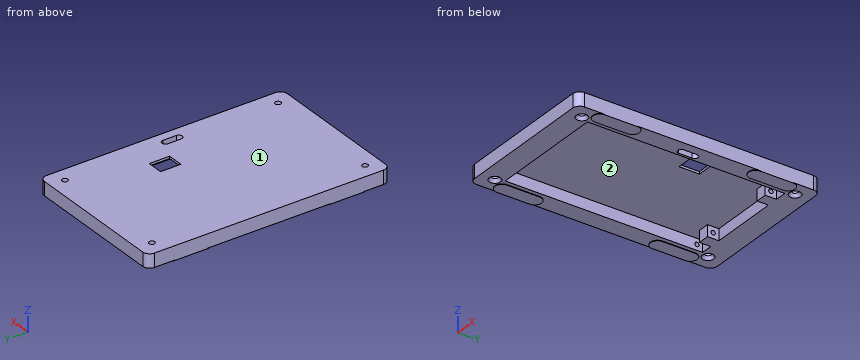
```python
from build123d import *

# Parameters (mm, degrees)
SKICA1_W                 = 67
SKICA1_H                 = 107
P_IDAT_VYSUNUT_M1_DEPTH  = 6
ZAOBLIT1_R               = 3
SKICA2_R                 = 1.25
ODEBRAT_VYSUNUT_M1_DEPTH = 7
ZKOSEN_1_SIZE            = 1.25
SKICA4_W                 = 7
SKICA4_H                 = 9
ODEBRAT_VYSUNUT_M2_DEPTH = 7
SKICA7_W                 = 51
SKICA7_H                 = 87
ODEBRAT_VYSUNUT_M3_DEPTH = 5
SKICA8_W                 = 5
SKICA8_H                 = 5
P_IDAT_VYSUNUT_M2_DEPTH  = 5
SKICA9_R                 = 0.95
ODEBRAT_VYSUNUT_M4_DEPTH = 14
SKICA10_R                = 0.95
ODEBRAT_VYSUNUT_M5_DEPTH = 14
P_IDAT_VYSUNUT_M3_DEPTH  = 0.2


with BuildPart() as part:
    # Skica1 → Přidat vysunutím1 (new body)
    with BuildSketch(Plane.XY):
        with Locations((33.5, 53.5)):
            Rectangle(SKICA1_W, SKICA1_H)
    extrude(amount=P_IDAT_VYSUNUT_M1_DEPTH)

    # Zaoblit1
    zaoblit1_edges = [part.edges().sort_by_distance(p)[0] for p in [
        (0, 107, 3),
        (67, 107, 3),
        (67, 0, 3),
        (0, 0, 3),
    ]]
    fillet(zaoblit1_edges, radius=ZAOBLIT1_R)

    # Skica2 → Odebrat vysunutím1 (cut, through all)
    with BuildSketch(Plane(origin=(0, 0, 0), x_dir=(-1, 0, 0), z_dir=(0, 0, -1))):
        with Locations((-6.5, 100.5)):
            Circle(SKICA2_R)
        with Locations((-60.5, 100.5)):
            Circle(SKICA2_R)
        with Locations((-6.5, 6.5)):
            Circle(SKICA2_R)
        with Locations((-60.5, 6.5)):
            Circle(SKICA2_R)
    extrude(amount=-ODEBRAT_VYSUNUT_M1_DEPTH, mode=Mode.SUBTRACT)

    # Zkosení1
    zkosen_1_edges = [part.edges().sort_by_distance(p)[0] for p in [
        (61.75, 100.5, 0),
        (7.75, 6.5, 0),
        (61.75, 6.5, 0),
        (7.75, 100.5, 0),
    ]]
    chamfer(zkosen_1_edges, length=ZKOSEN_1_SIZE)

    # Skica4 → Odebrat vysunutím2 (cut, through all)
    with BuildSketch(Plane(origin=(0, 0, 0), x_dir=(-1, 0, 0), z_dir=(0, 0, -1))):
        with Locations((-49, 64.5)):
            Rectangle(SKICA4_W, SKICA4_H)
        with BuildLine():
            Line((-60, 55.5), (-60, 49.55))
            ThreePointArc((-60, 49.55), (-61.5, 48.05), (-63, 49.55))
            Line((-63, 49.55), (-63, 55.5))
            ThreePointArc((-63, 55.5), (-61.5, 57), (-60, 55.5))
        make_face()
    extrude(amount=-ODEBRAT_VYSUNUT_M2_DEPTH, mode=Mode.SUBTRACT)

    # Skica7 → Odebrat vysunutím3 (cut)
    with BuildSketch(Plane(origin=(0, 0, 0), x_dir=(-1, 0, 0), z_dir=(0, 0, -1))):
        with Locations((-33.5, 53.5)):
            Rectangle(SKICA7_W, SKICA7_H)
    extrude(amount=-ODEBRAT_VYSUNUT_M3_DEPTH, mode=Mode.SUBTRACT)

    # Skica8 → Přidat vysunutím2 (add)
    with BuildSketch(Plane(origin=(0, 0, 5), x_dir=(-1, 0, 0), z_dir=(0, 0, -1))):
        with Locations((-51.4, 94.5)):
            Rectangle(SKICA8_W, SKICA8_H)
        with Locations((-15.6, 94.5)):
            Rectangle(SKICA8_W, SKICA8_H)
    extrude(amount=P_IDAT_VYSUNUT_M2_DEPTH)

    # Skica9 → Odebrat vysunutím4 (cut)
    with BuildSketch(Plane.ZY.offset(-48.9)):
        with Locations((2.5, 94.5)):
            Circle(SKICA9_R)
    extrude(amount=-ODEBRAT_VYSUNUT_M4_DEPTH, mode=Mode.SUBTRACT)

    # Skica10 → Odebrat vysunutím5 (cut)
    with BuildSketch(Plane(origin=(18.1, 0, 0), x_dir=(0, 0, -1), z_dir=(1, 0, 0))):
        with Locations((-2.5, 94.5)):
            Circle(SKICA10_R)
    extrude(amount=-ODEBRAT_VYSUNUT_M5_DEPTH, mode=Mode.SUBTRACT)

    # Skica11 → Přidat vysunutím3 (add)
    with BuildSketch(Plane(origin=(0, 0, 0), x_dir=(-1, 0, 0), z_dir=(0, 0, -1))):
        with BuildLine():
            Line((0, 95), (0, 80.6))
            ThreePointArc((0, 80.6), (-3.1, 77.5), (-6.2, 80.6))
            Line((-6.2, 80.6), (-6.2, 95))
            ThreePointArc((-6.2, 95), (-3.1, 98.1), (0, 95))
        make_face()
        with BuildLine():
            Line((0, 26.4), (0, 12))
            ThreePointArc((0, 12), (-3.1, 8.9), (-6.2, 12))
            Line((-6.2, 12), (-6.2, 26.4))
            ThreePointArc((-6.2, 26.4), (-3.1, 29.5), (0, 26.4))
        make_face()
        with BuildLine():
            Line((-60.8, 95), (-60.8, 80.6))
            ThreePointArc((-60.8, 80.6), (-63.9, 77.5), (-67, 80.6))
            Line((-67, 80.6), (-67, 95))
            ThreePointArc((-67, 95), (-63.9, 98.1), (-60.8, 95))
        make_face()
        with BuildLine():
            Line((-60.8, 26.4), (-60.8, 12))
            ThreePointArc((-60.8, 12), (-63.9, 8.9), (-67, 12))
            Line((-67, 12), (-67, 26.4))
            ThreePointArc((-67, 26.4), (-63.9, 29.5), (-60.8, 26.4))
        make_face()
    extrude(amount=P_IDAT_VYSUNUT_M3_DEPTH)


solid = part.part
```
Part model, mm, in its own coordinate system. Face numbers are marked on the shaded views. Round coordinates to 2 decimals unless told otherwise and drop trailing zeros. Loops run counter-clockwise (first coordinate to the right, second up) from the corner with the lowest first, then second, coordinate; pieces in that order, holes last. Notation, with made-up numbers: (3, -34) -> (41, -34) arc R21 ccw to (41, -26) -> close; hole circle Ø11 at (79, 72). An arc over 180 degrees is marked (long way). Use CSV: the item, a comma, the result in double quotes. Start each with the question number.
1) Cut at B-B, the plane z = 2.5. Give the number of separate pieces and of enclosed holes in the cut face, plus the area to 3 significant figures.
2) Cut at C-C, the plane y = 6.5. Write the cut outline in (x, z).
3) Drop flat-ended pins along their axis: P1, Ø1.5, axis at x = 60.5, y = 6.5, coming from the -Z side; P2, Ø3, axis at x = 58, y = 60.5, coming from the -Z side; P3, Ø4, axis at x = 6.5, y = 6.5, coming from the -Z side. Give the stop position or say it passes through.
4) Wall check: L1, parallel to X at y = 100.5, z = 3.45; L2, parallel to Y at x = 50.6, z = 2.5; L3, parallel to X at y = 55.5, z = 4. Give the ranges that are in metal, low to high. Write a range as [from, to].
5) Cut at D-D, the plane x = 27.5. Write the cut outline in (y, z).
6) Pull direction X, two halves, no side cores. Call the marked faces 1 and 2: +X half, -X half, draft (parallel to the pull), parting line (faces both ways), or undercut.
7) Cut at A-A, the plane y = 66.5. Write the cut outline in (x, z).
Determined:
1,separate pieces,"3"
1,enclosed holes,"6"
1,area,"2,700 mm2"
2,outline,"(0, 0) -> (4, 0) -> (5.25, 1.25) -> (5.25, 6) -> (0, 6) -> close; (7.75, 1.25) -> (9, 0) -> (58, 0) -> (59.25, 1.25) -> (59.25, 6) -> (7.75, 6) -> close; (61.75, 1.25) -> (63, 0) -> (67, 0) -> (67, 6) -> (61.75, 6) -> close"
3,P1,"passes through"
3,P2,"stops at z = 0"
3,P3,"stops at z = 0.5"
4,L1,"x = [0, 5.25], [7.75, 59.25], [61.75, 67]"
4,L2,"y = [0, 10], [92, 93.55], [95.45, 107]"
4,L3,"x = [0, 8], [59, 60], [63, 67]"
5,outline,"(0, 0) -> (10, 0) -> (10, 5) -> (97, 5) -> (97, 0) -> (107, 0) -> (107, 6) -> (0, 6) -> close"
6,face 1,"draft"
6,face 2,"undercut"
7,outline,"(0, 0) -> (8, 0) -> (8, 5) -> (45.5, 5) -> (45.5, 6) -> (0, 6) -> close; (52.5, 5) -> (59, 5) -> (59, 0) -> (67, 0) -> (67, 6) -> (52.5, 6) -> close"
